Geometry: see drawing. Coordinates: mm, zero at the bounding-box minimum. A direction names the side the tool comes from. Coordinates: 2 decimals unless noted, no trailing zeros. Loops run counter-clockwise (first coordinate to the right, second up) from the corner with the lowest first, then second, coordinate; pieces in that order, holes last. Notation, with made-up numbers: (55.5, 75.5) - (108.5, 75.5) arc R12 ccw to (108.5, 83.5) - close; hole circle Ø3 at (8, -27.75). An arc over 180 degrees is marked (long way). Answer in a Markdown table with one row per item.
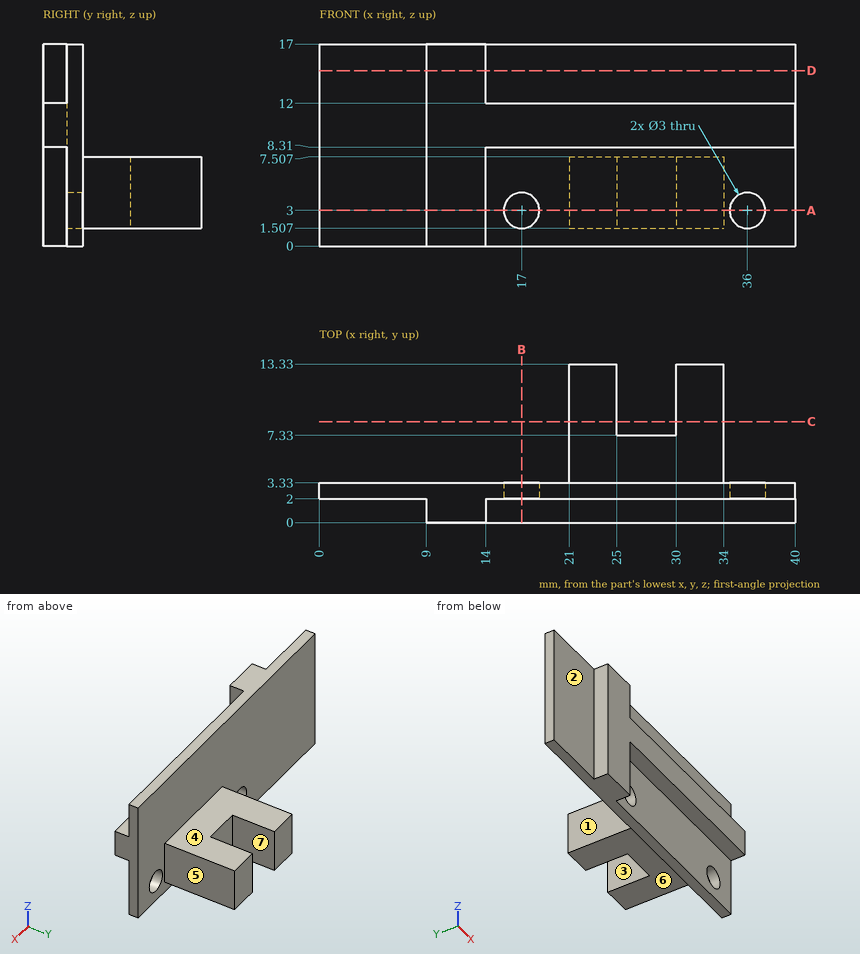
(1) Cut plane A-A on z = 3. Output: boundary loops of the cut face in (x, y), then the cut area to 3 significant figures.
Verdict:
| item | result |
|---|---|
| outline | (0, 2) - (9, 2) - (9, 0) - (14, 0) - (14, 2) - (15.5, 2) - (15.5, 3.33) - (0, 3.33) - close; (18.5, 2) - (34.5, 2) - (34.5, 3.33) - (34, 3.33) - (34, 13.33) - (30, 13.33) - (30, 7.33) - (25, 7.33) - (25, 13.33) - (21, 13.33) - (21, 3.33) - (18.5, 3.33) - close; (37.5, 2) - (40, 2) - (40, 3.33) - (37.5, 3.33) - close |
| area | 155 mm² |
(2) Ray query, probe 1 along X at (y, z) = (2.95, 3); probe 2 along X at (y, z) = (11.5, 2.25); probe 3 along Y at (x, z) = (22.5, 14.5). Return the intervals inside material, ascending.
Verdict:
| item | result |
|---|---|
| probe 1 | x = 0 to 15.5, 18.5 to 34.5, 37.5 to 40 |
| probe 2 | x = 21 to 25, 30 to 34 |
| probe 3 | y = 2 to 3.33 |
(3) Cut plane B-B on x = 17. Output: boundary loops of the cut face in (y, z).
Verdict:
| item | result |
|---|---|
| outline | (0, 8.31) - (2, 8.31) - (2, 4.5) - (3.33, 4.5) - (3.33, 17) - (2, 17) - (2, 12) - (0, 12) - close; (2, 0) - (3.33, 0) - (3.33, 1.5) - (2, 1.5) - close |
(4) Access query for the marked faces 4, 5, 6 and 7. Directions: +Z, -Z, +X, -X, +Y, -Y. A direction counts if a zero-diameter tool reaches every point of the face in a straight line with its end or side. Return the directions, or none.
Verdict:
| item | result |
|---|---|
| face 4 | +Z, +X, -X, +Y |
| face 5 | +Z, -Z, +X, +Y |
| face 6 | -Z, +X, -X, +Y |
| face 7 | +Z, -Z, +Y |
(5) First-contact query: pin 1 Ø4.5 at (x, z) = (4, 10.5) entering from -Y; pin 2 Ø5 at (y, z) = (10, 6) entering from -X; pin 3 Ø3 at (x, y) = (30, 8) entering from -Z; pin 4 Ø1.8 at (x, z) = (17, 3) entering from -Y. Flat tips, straight axial feed; report the tip coordinate or a pass-through.
Verdict:
| item | result |
|---|---|
| pin 1 | stops at y = 2 |
| pin 2 | stops at x = 21 |
| pin 3 | stops at z = 1.51 |
| pin 4 | passes through |
(6) Pull-direction query (X, two-part tool) for the marked faces 1, 2 and 3; classes: pulls with the +X half, pulls with the -X half, needs draft (parallel to the pull), parting line crosses it, or undercut.
Verdict:
| item | result |
|---|---|
| face 1 | pulls with the -X half |
| face 2 | needs draft |
| face 3 | undercut |
(7) Cut plane D-D on z = 14.75. Output: boundary loops of the cut face in (x, y).
Verdict:
| item | result |
|---|---|
| outline | (0, 2) - (9, 2) - (9, 0) - (14, 0) - (14, 2) - (40, 2) - (40, 3.33) - (0, 3.33) - close |
(8) Cut plane C-C on y = 8.5. Output: boundary loops of the cut face in (x, z).
Verdict:
| item | result |
|---|---|
| outline | (21, 1.51) - (25, 1.51) - (25, 7.51) - (21, 7.51) - close; (30, 1.51) - (34, 1.51) - (34, 7.51) - (30, 7.51) - close |
